Geometry: final body of the model. Coordinates: model frame, mm. Give positions to 0.01 mm unless a question says otherwise; leave off trailing zeros. Order: outer loops, then holes, each group sorted by start corner. A loop starts at its lowest first (then second) coordinate and runs counter-clockwise, first axis right, second up. Notation, with made-up numbers: (13.25, 53) - (61.25, 53) arc R34 ccw to (61.25, 83) - close; hole circle Ø10 at (-10, -18.75). An arc over 180 degrees is marked (long way). Write item = value, one per line. Start each with the question number.
Autodesk Inventor part; units mm, degrees
ref_plane "YZ Plane" through (0, 0, 0) normal (1, 0, 0) x (0, 1, 0)
ref_plane "XZ Plane" through (0, 0, 0) normal (0, 1, 0) x (-1, 0, 0)
ref_plane "XY Plane" through (0, 0, 0) normal (0, 0, 1) x (1, 0, 0)
sketch "草图1" plane through (0, 0, 0) normal (1, 0, 0) x (0, 1, 0)
  circle A0 centre (0, 0) radius 61
  circle A1 centre (0, 0) radius 37
  circle A2 centre (48.5, 0) radius 5.5
  circle A3 centre (0, 48.5) radius 5.5
  circle A4 centre (-48.5, 0) radius 5.5
  circle A5 centre (0, -48.5) radius 5.5
  dimension "d1" = 122
  dimension "d3" = 74
  dimension "d4" = 11
  dimension "d5" = 48.5
  dimension "d8" = 360
extrude "拉伸1" add sketch "草图1" along normal blind 0.5
equation "\"d1\" = D2"
equation "\"d3\" = d2"
equation "\"d4\" = d0"
equation "\"d10\" = b"
equation "\"b\" = 0.5"
equation "\"d0\" = 11"
equation "\"D0\" = 97"
equation "\"d2\" = 74"
equation "\"D2\" = 122"
properties part number "中间轴承调整垫片" material "铜，锻铸"
Q1. Section C-C, the plane z = -13. Return the cut outline in (x, y).
Q2. Material intervals for line 1 along Z through (x, y) = (0.45, 0); line 2 along Z through (x, y) = (0.15, -48.5); line 3 along Y through (x, z) = (0.1, -5), sorted ascending. Write a range as from..to.
Q3. Section A-A, the plane y = 0. Return the cut outline in (x, z).
Q4. Pull-direction query (Z, two-part tool) for faces 1 (the cylindrical face through (0.246, -0.716, -53.953)), 2 (the flat face through (0, 26.3, -26.3)), 3 (the cylindrical face through (0.246, -48.408, 37.118)); classes: +Z half, -Z half, draft (parallel to the pull), parting line (faces both ways), or undercut.
Q5. Contact query for a flat-ended pin moving along its axis: pin 1 (6.5 mm diameter, centred on y = 0, z = 48.5, fed in from +X). Output: stop coordinate, or through.
Q6. Section D-D, the plane y = 33. Return the cut outline in (x, z).
Q7. Section B-B, the plane x = 0.4. Return the cut outline in (y, z), then the cut area to 3 significant figures.
The answers:
q1.outline = (0, -59.6) - (0.5, -59.6) - (0.5, -34.64) - (0, -34.64) - close; (0, 34.64) - (0.5, 34.64) - (0.5, 59.6) - (0, 59.6) - close
q2.line_1 = -61..-54, -43..-37, 37..43, 54..61
q2.line_2 = -37..-5.5, 5.5..37
q2.line_3 = -60.79..-50.79, -46.21..-36.66, 36.66..46.21, 50.79..60.79
q3.outline = (0, -61) - (0.5, -61) - (0.5, -54) - (0, -54) - close; (0, -43) - (0.5, -43) - (0.5, -37) - (0, -37) - close; (0, 37) - (0.5, 37) - (0.5, 43) - (0, 43) - close; (0, 54) - (0.5, 54) - (0.5, 61) - (0, 61) - close
q4.face_1 = undercut
q4.face_2 = draft
q4.face_3 = parting line
q5.pin_1 = through
q6.outline = (0, -51.3) - (0.5, -51.3) - (0.5, -16.73) - (0, -16.73) - close; (0, 16.73) - (0.5, 16.73) - (0.5, 51.3) - (0, 51.3) - close
q7.outline = circle Ø122 at (0, 0); hole circle Ø11 at (-48.5, 0); hole circle Ø74 at (0, 0); hole circle Ø11 at (0, -48.5); hole circle Ø11 at (0, 48.5); hole circle Ø11 at (48.5, 0)
q7.area = 7,010 mm²
